Geometry check sheet. Reference: the model listing, model coordinates, mm. Coordinates: 2 decimals unless noted, no trailing zeros. Order: outer loops, then holes, each group sorted by start corner. A loop starts at its lowest first (then second) coordinate and runs counter-clockwise, first axis right, second up. Notation, with made-up numbers: (70.5, -22.5) - (76.5, -22.5) arc R8 cw to (76.5, -15.5) - close; hole circle Ø2 at (65, 46). An arc over 180 degrees is marked (long way). Return JSON: item names as keys, results as strings. Group by question number.
Item 1: Section check A-A on y = 9.75. Enter the section's corners in (x, z), then the cut area to 3 significant figures.
Item 2: Gauge pin test, flat ends, axial feed: pin 1 (6 mm diameter, centred on x = 8, y = 12.5, fed in from +Z); pin 2 (8 mm diameter, centred on y = 9.5, z = 10, fed in from -X). Record the tip position at first contact, or that the pin passes through.
Item 3: Scan lines: probe 1 along X at (y, z) = (15.5, -0.25); probe 2 along X at (y, z) = (4, 2.5); probe 3 along Z at (x, y) = (11.75, 13.25). Record each from-to range of solid material in increasing order.
Item 4: Section check B-B on y = 17. Enter the section's corners in (x, z), then the cut area to 3 significant figures.
from build123d import *

# Parameters (mm, degrees)
F0_R     = 13.97
F1_DEPTH = 19.05
F2_R     = 2.54


# Not quite as in the source:
# - a feature names something its author has since deleted; it is built from what else it names


with BuildPart() as f1:
    # F0 (on Front) → F1 (new body)
    with BuildSketch(Plane.XZ):
        with Locations((-63.3578656336, 0)):
            Circle(F0_R)
    extrude(amount=-F1_DEPTH)

    # F2
    f2_edges = [f1.edges().sort_by_distance(p)[0] for p in [
        (-77.327866, 19.05, 0),
    ]]
    fillet(f2_edges, radius=F2_R)


with BuildPart() as f1_1:
    # F3: moved
    add(f1.part.moved(Location((65.786, 0, 0))))


solid = f1_1.part
Computed:
{
 "1": {"outline": "circle Ø27.94 at (2.43, 0)", "area": "613 mm²"},
 "2": {"pin 1": "stops at z = 13.73", "pin 2": "stops at x = -10.19"},
 "3": {"probe 1": "x = -11.54 to 16.4", "probe 2": "x = -11.32 to 16.17", "probe 3": "z = -10.4 to 10.4"},
 "4": {"outline": "circle Ø27.84 at (2.43, 0)", "area": "609 mm²"}
}
